Geometry check sheet. Reference: drawing and pictorial views, mm from the part's lowest x, y, z. Round coordinates to 2 decimals unless told otherwise and drop trailing zeros. Order: outer loops, then holes, each group sorted by start corner. A loop starts at its lowest first (then second) coordinate and runs counter-clockwise, first axis right, second up.
(1) Sectioned sample at C-C, the plane z = 3.25. Enter the section's corners in (x, y), and give its area (3 significant figures).
(2) Sectioned sample at B-B, the plane x = 114. Enter the section's corners in (y, z), and give its area (3 significant figures).
(3) Sectioned sample at A-A, the plane y = 357.5. Enter the section's corners in (x, z).
(4) Thickness scan on probe 1 along Y at (x, z) = (230.5, 3); probe 2 along X at (y, z) = (372, 2.25). Record the ranges inside material, lowest first.
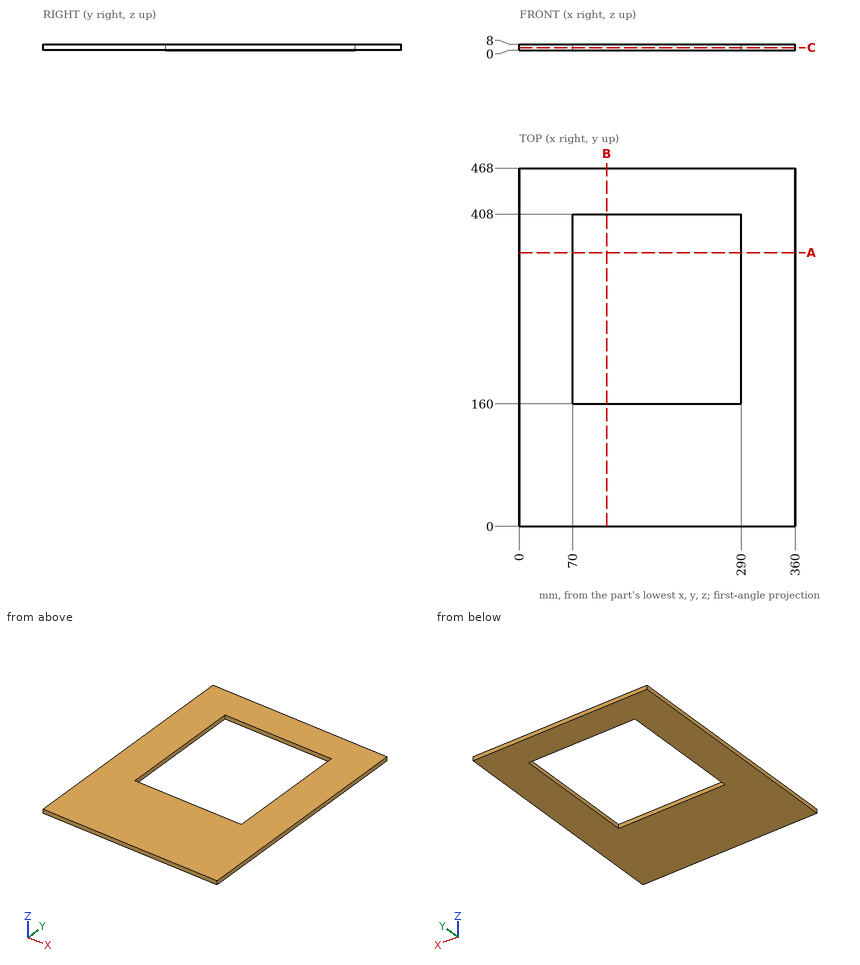
Derived:
1. outline: (0, 0) - (360, 0) - (360, 468) - (0, 468) - close; hole (70, 160) - (290, 160) - (290, 408) - (70, 408) - close
1. area: 114,000 mm2
2. outline: (0, 0) - (160, 0) - (160, 8) - (0, 8) - close; (408, 0) - (468, 0) - (468, 8) - (408, 8) - close
2. area: 1,760 mm2
3. outline: (0, 0) - (70, 0) - (70, 8) - (0, 8) - close; (290, 0) - (360, 0) - (360, 8) - (290, 8) - close
4. probe 1: y = 0 to 160, 408 to 468
4. probe 2: x = 0 to 70, 290 to 360
